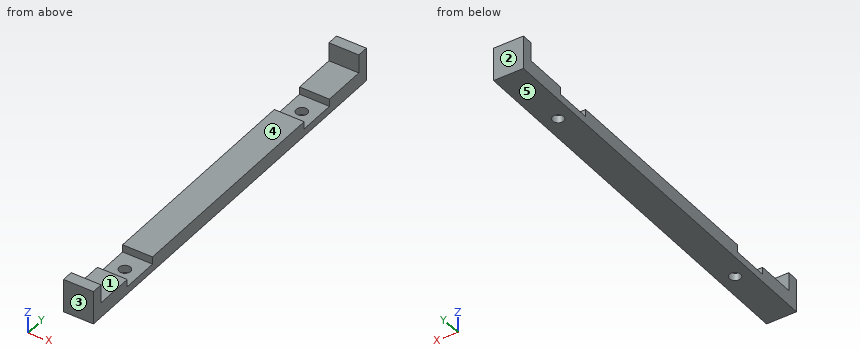
```python
from build123d import *

# Parameters (mm, degrees)
F0_W     = 8
F0_H     = 108
F1_DEPTH = 2
F2_W     = 8
F2_H     = 3
F3_DEPTH = 5
F5_D     = 3
F6_W     = 8
F6_H     = 10
F6_R     = 1.5
F7_DEPTH = 2


with BuildPart() as f1:
    # F0 (on Top) → F1 (new body, symmetric)
    with BuildSketch(Plane.XY):
        Rectangle(F0_W, F0_H)
    extrude(amount=F1_DEPTH, both=True)

    # F2 (on face) → F3 (join)
    with BuildSketch(Plane.XY.offset(2)):
        with Locations((0, 52.5)):
            Rectangle(F2_W, F2_H)
        with Locations((0, -52.5)):
            Rectangle(F2_W, F2_H)
    extrude(amount=F3_DEPTH)

    # F5 (through all)
    with Locations(Plane.XY.offset(2)):
        with Locations((0, 34.365942), (0, -35.634058)):
            Hole(F5_D / 2)

    # F6 (on face) → F7 (cut)
    with BuildSketch(Plane.XY.offset(2)):
        with Locations((0, -35.634058)):
            Rectangle(F6_W, F6_H)
        with Locations((0, -35.634058)):
            Circle(F6_R, mode=Mode.SUBTRACT)
        with Locations((0, 34.365942)):
            Rectangle(F6_W, F6_H)
        with Locations((0, 34.365942)):
            Circle(F6_R, mode=Mode.SUBTRACT)
    extrude(amount=-F7_DEPTH, mode=Mode.SUBTRACT)


solid = f1.part
```
Check sheet for the modelled part. Datum: model origin and axes. Units: mm. Face numbers are marked on the shaded views. A direction names the side the tool comes from. Round coordinates to 2 decimals unless told otherwise and drop trailing zeros. Order: outer loops, then holes, each group sorted by start corner. A loop starts at its lowest first (then second) coordinate and runs counter-clockwise, first axis right, second up. Notation, with made-up numbers: (20.5, 76) -> (50.5, 76) arc R18 cw to (50.5, 84) -> close; hole circle Ø4 at (-39.5, -38.5). An arc over 180 degrees is marked (long way). Use CSV: the item, a comma, the result in double quotes.
(1) Cross-section at C-C (y = 10.5). Record the boundary of the cut face in (x, z), and give its area (3 significant figures).
Worked out:
outline,"(-4, -2) -> (4, -2) -> (4, 2) -> (-4, 2) -> close"
area,"32.0 mm²"
(2) Cross-section at B-B (x = 0). Record the boundary of the cut face in (y, z).
Worked out:
outline,"(-54, -2) -> (-37.13, -2) -> (-37.13, 0) -> (-40.63, 0) -> (-40.63, 2) -> (-51, 2) -> (-51, 7) -> (-54, 7) -> close; (-34.13, -2) -> (32.87, -2) -> (32.87, 0) -> (29.37, 0) -> (29.37, 2) -> (-30.63, 2) -> (-30.63, 0) -> (-34.13, 0) -> close; (35.87, -2) -> (54, -2) -> (54, 7) -> (51, 7) -> (51, 2) -> (39.37, 2) -> (39.37, 0) -> (35.87, 0) -> close"
(3) Tool access check on the marked faces 1 and 2. Record the directions out of +Z, -Z, +X, -X, +Y, -Y that give a thin tool (end or side, any length) a straight path to the whole face; none if there is none.
Worked out:
face 1,"+Z, +X, -X"
face 2,"+Z, -Z, +X, -X, +Y"
(4) Draft check along Y on the marked faces 3, 4 and 5. Enter one of: pulls with the +Y half, pulls with the -Y half, needs draft (parallel to the pull), parting line crosses it, or undercut.
Worked out:
face 3,"pulls with the -Y half"
face 4,"undercut"
face 5,"needs draft"
(5) Cross-section at A-A (z = 5). Record the boundary of the cut face in (x, y), and give its area (3 significant figures).
Worked out:
outline,"(-4, -54) -> (4, -54) -> (4, -51) -> (-4, -51) -> close; (-4, 51) -> (4, 51) -> (4, 54) -> (-4, 54) -> close"
area,"48.0 mm²"
(6) Depth check by flat-ended pin: pin 1 (4 mm diameter, centred on x = 2, y = 1.5, fed in from +Z). Enter the tip coordinate at first touch or a pass-through.
Worked out:
pin 1,"z = 2"
(7) Material ranges on line 1 along Y through (x, z) = (1.75, 0.5); line 2 along Y through (x, z) = (0, -0.4); line 3 along Y through (x, z) = (0, 2.75), recorded low to high. Write a range as from..to.
Worked out:
line 1,"-54..-40.63, -30.63..29.37, 39.37..54"
line 2,"-54..-37.13, -34.13..32.87, 35.87..54"
line 3,"-54..-51, 51..54"
